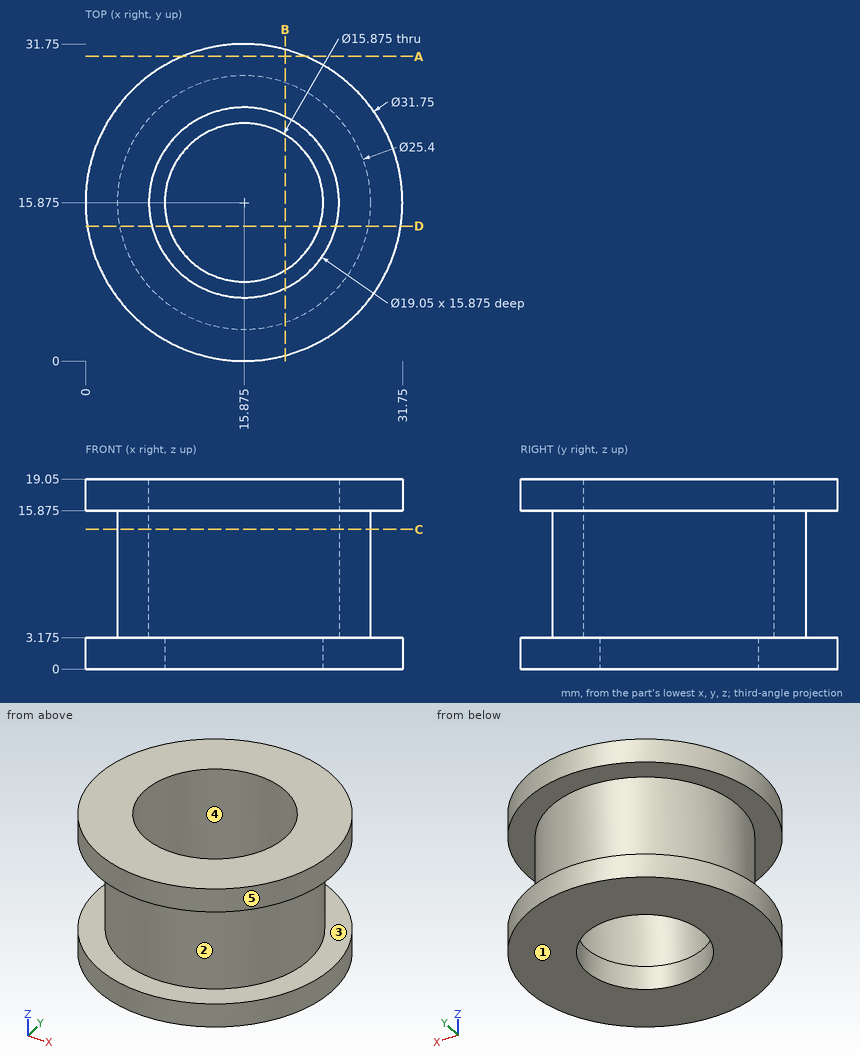
The figure shows three views and two pictorial views of one solid part (mm, origin at its lowest corner). Answer the questions. A direction names the side the tool comes from. Round coordinates to 2 decimals unless told otherwise and drop trailing zeros. Write each loop counter-clockwise with the first axis right and the second up, starting at its lowest first coordinate (ties: lowest second). Pieces come first, ordered by that corner, then holes. Notation, with made-up numbers: M 66.25,14 L 94.25,14 A12 cw 94.25,36 Z; hole C 70.25,52 d2. An arc over 180 degrees is marked long. Write each question's results on one line, items separated by ' | '. Start each with the question number.
(1) The part is cut by section A-A, the plane y = 30.5. Write down the section's boundary in (x, z) (3 decimals), and give its area (3 significant figures).
(2) Find the intervals of material crossed by line 1 (Z direction, x = 30.5, y = 10) (3 decimals); line 2 (Y direction, x = 16, z = 18.25); line 3 (Y direction, x = 16, z = 1.75), in increasing order.
(3) Determine the mould class of the marked faces 3, 4 and 5 for opening direction X: +X half, -X half, draft (parallel to the pull), parting line (faces both ways), or undercut.
(4) The part is cut by section C-C, the plane z = 14. Write down the section's boundary in (x, y) (3 decimals).
(5) For the marked faces 1 and 2, determine the directions among +Z, -Z, +X, -X, +Y, -Y from which every point of the face is accessible in a straight line to the end or side of a thin tool.
(6) The part is cut by section D-D, the plane y = 13.5. Write down the section's boundary in (x, z) (3 decimals).
(7) Each of these flat-tipped pins is pushed along its axis until it touches: P1, Ø10, axis at x = 16, y = 21, coming from the +Z side; P2, Ø2, axis at y = 10.5, z = 12.5, coming from the +X side; P3, Ø5, axis at y = 15, z = 8.5, coming from the -X side (3 decimals); P4, Ø1, axis at y = 22.5, z = 3.5, coming from the +X side. Where does it stop, or does it pass through?
(8) The part is cut by section B-B, the plane x = 20. Write down the section's boundary in (y, z) (3 decimals).
Worked answers:
1) outline: M 9.7,0 L 22.05,0 L 22.05,3.175 L 9.7,3.175 Z; M 9.7,15.875 L 22.05,15.875 L 22.05,19.05 L 9.7,19.05 Z | area: 78.4 mm²
2) line 1: z = 0 to 3.175, 15.875 to 19.05 | line 2: y = 0 to 6.35, 25.4 to 31.75 | line 3: y = 0 to 7.94, 23.81 to 31.75
3) face 3: draft | face 4: undercut | face 5: parting line
4) outline: C 15.875,15.875 d25.4; hole C 15.875,15.875 d19.05
5) face 1: -Z, +X, -X, +Y, -Y | face 2: none
6) outline: M 0.179,0 L 8.301,0 L 8.301,3.175 L 6.651,3.175 L 6.651,19.05 L 0.179,19.05 L 0.179,15.875 L 3.399,15.875 L 3.399,3.175 L 0.179,3.175 Z; M 23.449,0 L 31.571,0 L 31.571,3.175 L 28.351,3.175 L 28.351,15.875 L 31.571,15.875 L 31.571,19.05 L 25.099,19.05 L 25.099,3.175 L 23.449,3.175 Z
7) P1: stops at z = 19.05 | P2: stops at x = 27.8 | P3: stops at x = 3.175 | P4: stops at x = 30.47
8) outline: M 0.545,0 L 9.094,0 L 9.094,3.175 L 7.29,3.175 L 7.29,19.05 L 0.545,19.05 L 0.545,15.875 L 3.864,15.875 L 3.864,3.175 L 0.545,3.175 Z; M 22.656,0 L 31.205,0 L 31.205,3.175 L 27.886,3.175 L 27.886,15.875 L 31.205,15.875 L 31.205,19.05 L 24.46,19.05 L 24.46,3.175 L 22.656,3.175 Z
